Autodesk Fusion 360 part; units mm, degrees
sketch "Sketch1" plane through (0, 0, 0) normal (0, 0, 1) x (1, 0, 0)
  circle A0 centre (0, 0) radius 7.5
  dimension "d1" = 15
extrude "Extrude1" add sketch "Sketch1" along normal blind 30
sketch "Sketch2" plane through (0, 0, 30) normal (0, 0, 1) x (-1, 0, 0)
  circle A0 centre (0, 0) radius 7.5
  line L0 (0, 0) -> (-10.0601, 0)
  line L1 (-10.0601, 0) -> (-10.0601, -9.4901)
  line L2 (-10.0601, -9.4901) -> (0, -9.4901)
  line L3 (0, -9.4901) -> (0, 0)
sketch "Sketch3" plane through (0, 0, 30) normal (0, 0, 1) x (-1, 0, 0)
  circle A0 centre (0, 0) radius 7.5
  circle A1 centre (0, 0) radius 5
  dimension "d8" = 10
extrude "Extrude4" cut sketch "Sketch3" against normal blind 2 contours A1
sketch "Sketch4" plane through (0, 0, 28) normal (0, 0, 1) x (-1, 0, 0)
  circle A0 centre (0, 0) radius 5
  circle A1 centre (0, 0) radius 3
  dimension "d11" = 6
extrude "Extrude5" cut sketch "Sketch4" against normal blind 2 contours A1
sketch "Sketch5" plane through (0, 0, 26) normal (0, 0, 1) x (-1, 0, 0)
  circle A0 centre (0, 0) radius 3
  line L0 (-8, -8) -> (5, -8)
  line L1 (5, -8) -> (5, 5)
  line L2 (5, 5) -> (-8, 5)
  line L3 (-8, 5) -> (-8, -8)
  line L4 (-8, -8) -> (5, 5) construction
  line L5 (5, -8) -> (-8, 5) construction
  point P0 (-1.5, -1.5)
extrude "Extrude6" cut sketch "Sketch5" against normal blind 7 contours A0 | L0 L1 L2 L3
sketch "Sketch6" plane through (0, 0, 19) normal (0, 0, 1) x (-1, 0, 0)
  arc A0 (-5.5902, 5) -> (5, -5.5902) centre (0, 0) ccw
  line L0 (5, -5.5902) -> (5, 5)
  line L1 (5, 5) -> (-5.5902, 5)
  circle A1 centre (0, 0) radius 3
  dimension "d16" = 6
extrude "Extrude7" cut sketch "Sketch6" against normal blind 10 contours A1
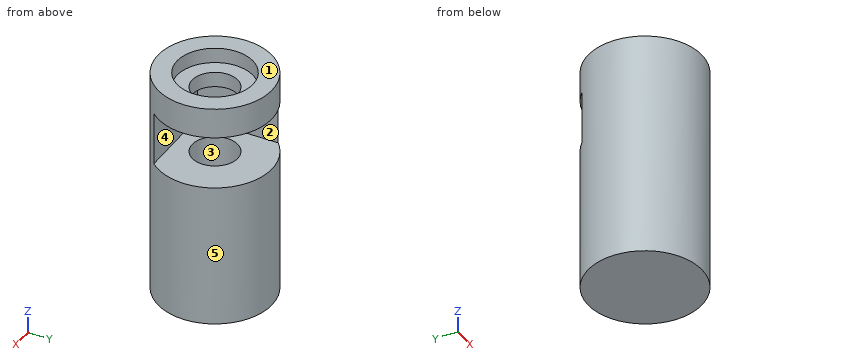
Design review of the part built by this model. Coordinates are the model's own, in mm. Face numbers are marked on the shaded views. A direction names the side the tool comes from. Coordinates: 2 decimals unless noted, no trailing zeros. Write each loop counter-clockwise with the first axis right and the second up, starting at its lowest first coordinate (ties: lowest second). Pieces come first, ordered by that corner, then holes. Notation, with made-up numbers: (-27, 28) - (28, 28) arc R7 cw to (28, 39) - close; hole circle Ø10 at (79, 25.25). An arc over 180 degrees is marked (long way). One line per item, written item: value.
1) Add section A-A (x = 0). State the section outline as (y, z) points, plus the area to 4 significant figures.
Answer sheet:
outline: (-7.5, 0) - (7.5, 0) - (7.5, 19) - (3, 19) - (3, 9) - (-3, 9) - (-3, 19) - (-5, 19) - (-5, 26) - (-3, 26) - (-3, 28) - (-5, 28) - (-5, 30) - (-7.5, 30) - close; (3, 26) - (7.5, 26) - (7.5, 30) - (5, 30) - (5, 28) - (3, 28) - close
area: 270.5 mm2
2) Add section D-D (y = 6.25). State the section outline as (x, z) points, plus the area to 3 significant figures.
Answer sheet:
outline: (-4.15, 0) - (4.15, 0) - (4.15, 19) - (-4.15, 19) - close; (-4.15, 26) - (4.15, 26) - (4.15, 30) - (-4.15, 30) - close
area: 191 mm2
3) Add section C-C (z = 12.5). State the section outline as (x, y) points.
Answer sheet:
outline: circle Ø15 at (0, 0); hole circle Ø6 at (0, 0)
4) Mouldability with a two-part tool opening along Z and no side actions: class the marked faces 1, 2 and 3 as +Z half, -Z half, draft (parallel to the pull), parting line (faces both ways), or undercut.
Answer sheet:
face 1: +Z half
face 2: undercut
face 3: draft
5) Insertion check: pin 1 (1.5 mm diameter, centred on y = -5.5, z = 23, fed in from -X); pin 2 (1.5 mm diameter, centred on x = -3.5, z = 16.5, fed in from -Y); pin 3 (5 mm diameter, centred on x = 0, y = 0, fed in from +Z); pin 4 (3 mm diameter, centred on x = -3.5, y = -2, fed in from -Z). Each pin has a flat end and moves straight along its axis. Give the tip position at first contact, or say it passes through.
Answer sheet:
pin 1: stops at x = -5.8
pin 2: stops at y = -6.98
pin 3: stops at z = 9
pin 4: stops at z = 0
6) For the marked faces 4 and 5, list the 3-axis set-ups (+Z, -Z, +X, -X, +Y, -Y) from which the entire face can be reached by the end or side of a thin tool; tool diameter is ignored.
Answer sheet:
face 4: +X, +Y
face 5: +Z, -Z
7) To check wall thickness, follow probe 1 along Z at (x, y) = (4.75, -2.5); probe 2 along Y at (x, z) = (0, 28.6); probe 3 along Z at (x, y) = (4.5, 2). State the ranges of each line that lie inside material, in increasing order.
Answer sheet:
probe 1: z = 0 to 19, 26 to 30
probe 2: y = -7.5 to -5, 5 to 7.5
probe 3: z = 0 to 19, 26 to 28
